from build123d import *

# Parameters (mm, degrees)
SALIENTE_EXTRUIR1_DEPTH = 15
CROQUIS5_R              = 2.575
CORTAR_EXTRUIR1_DEPTH   = 4


with BuildPart() as part:
    # Croquis2 → Saliente-Extruir1 (new body)
    with BuildSketch(Plane(origin=(0, 0, 0), x_dir=(0, 0, -1), z_dir=(1, 0, 0))):
        Polygon((-22.95, -12.8), (-9.95, -12.8), (-9.95, -3), (9.95, -3), (9.95, -12.8), (22.95, -12.8), (22.95, -9.8), (12.95, -9.8), (12.95, 0), (-12.95, 0), (-12.95, -9.8), (-22.95, -9.8), align=None)
    extrude(amount=SALIENTE_EXTRUIR1_DEPTH)

    # Croquis5 → Cortar-Extruir1 (cut, through all)
    with BuildSketch(Plane(origin=(0, -9.8, 0), x_dir=(1, 0, 0), z_dir=(0, 1, 0))):
        with Locations((7.5, -17.95)):
            Circle(CROQUIS5_R)
    cortar_extruir1 = extrude(amount=-CORTAR_EXTRUIR1_DEPTH, mode=Mode.SUBTRACT)

    # Simetría1: Cortar-Extruir1 across plane
    add(cortar_extruir1.mirror(Plane.XY), mode=Mode.SUBTRACT)


solid = part.part
The listing builds one solid part. Answer for the finished solid, in the listing's coordinates (mm). A direction names the side the tool comes from. Round coordinates to 2 decimals unless told otherwise and drop trailing zeros. Write each loop counter-clockwise with the first axis right and the second up, starting at its lowest first coordinate (ties: lowest second). Pieces come first, ordered by that corner, then holes. Notation, with made-up numbers: (-32.75, 29.5) - (-25.75, 29.5) arc R32 ccw to (-25.75, 67.5) - close; hole circle Ø7 at (43, 84.5). An arc over 180 degrees is marked (long way). Use one line per item in the form item = value. Start each with the question number.
Item 1: A cutting plane is placed at C-C (z = 17.95). Write down the section's boundary in (x, y) (3 decimals).
Item 2: Flat-ended cylindrical pins translate along their axes: pin 1 Ø6.5 at (x, z) = (7.5, -17.95) entering from +Y; pin 2 Ø1 at (x, z) = (10.5, 3) entering from -Y; pin 3 Ø5 at (x, y) = (9.5, -6) entering from -Z. Find the tip coordinate at first contact, or state that the pin passes through.
Item 3: A cutting plane is placed at D-D (y = -8.25). Write down the section's boundary in (x, z), plus the area to 3 significant figures.
Item 4: A cutting plane is placed at B-B (x = 7.5). Write down the section's boundary in (y, z) (3 decimals).
Item 5: A cutting plane is placed at A-A (y = -10.5). Write down the section's boundary in (x, z) (3 decimals).
Item 6: Determine the mould class of faces 5 (the flat face through (7, -11, 22.95)), 6 (the flat face through (7, -5, -12.95)), 7 (the flat face through (7, -3, 0)), 8 (the flat face through (15, -2.6, -1.6)) for opening direction Z: +Z half, -Z half, draft (parallel to the pull), parting line (faces both ways), or undercut.
Item 7: Find the intervals of material crossed by line 1 (Z direction, x = 7.5, y = -11.9) (3 decimals); line 2 (Z direction, x = 6.75, y = -5); line 3 (X direction, y = -10.65, z = 17.95) (3 decimals), in increasing order. Write a range as [from, to].
Item 8: A tool of negligible diameter and unlimited length cuts with its end or side. For faces 1 (the flat face through (7, -5, 12.95)), 2 (the flat face through (0, -2.6, -1.6)), 3 (the flat face through (9.1, -9.8, -20.2)), 4 (the flat face through (7, -8, 9.95)), from which of +Z, -Z, +X, -X, +Y, -Y can it reach the whole face along a straight path? Write none if from no direction.
The answers:
q1.outline = (0, -12.8) - (4.925, -12.8) - (4.925, -9.8) - (0, -9.8) - close; (10.075, -12.8) - (15, -12.8) - (15, -9.8) - (10.075, -9.8) - close
q2.pin_1 = -9.8
q2.pin_2 = -3
q2.pin_3 = -12.95
q3.outline = (0, -12.95) - (15, -12.95) - (15, -9.95) - (0, -9.95) - close; (0, 9.95) - (15, 9.95) - (15, 12.95) - (0, 12.95) - close
q3.area = 90.0 mm^2
q4.outline = (-12.8, -22.95) - (-9.8, -22.95) - (-9.8, -20.525) - (-12.8, -20.525) - close; (-12.8, -15.375) - (-9.8, -15.375) - (-9.8, -12.95) - (0, -12.95) - (0, 12.95) - (-9.8, 12.95) - (-9.8, 15.375) - (-12.8, 15.375) - (-12.8, 9.95) - (-3, 9.95) - (-3, -9.95) - (-12.8, -9.95) - close; (-12.8, 20.525) - (-9.8, 20.525) - (-9.8, 22.95) - (-12.8, 22.95) - close
q5.outline = (0, -22.95) - (15, -22.95) - (15, -9.95) - (0, -9.95) - close; (0, 9.95) - (15, 9.95) - (15, 22.95) - (0, 22.95) - close; hole circle Ø5.15 at (7.5, -17.95); hole circle Ø5.15 at (7.5, 17.95)
q6.face_5 = +Z half
q6.face_6 = -Z half
q6.face_7 = undercut
q6.face_8 = draft
q7.line_1 = [-22.95, -20.525], [-15.375, -9.95], [9.95, 15.375], [20.525, 22.95]
q7.line_2 = [-12.95, -9.95], [9.95, 12.95]
q7.line_3 = [0, 4.925], [10.075, 15]
q8.face_1 = +Z, +X, -X, +Y
q8.face_2 = +Z, -Z, -X, +Y, -Y
q8.face_3 = -Z, +X, -X, +Y
q8.face_4 = +X, -X, -Y
